The listing builds one solid part. Answer for the finished solid, in the listing's coordinates (mm). A direction names the side the tool comes from. Round coordinates to 2 decimals unless told otherwise and drop trailing zeros. Write each loop counter-clockwise with the first axis right and the second up, starting at its lowest first coordinate (ties: lowest second). Pieces come first, ordered by that corner, then holes. Notation, with made-up numbers: (85.25, 26) - (123.25, 26) arc R21 ccw to (123.25, 56) - close; hole circle Ø5 at (-21, 50.5). An arc over 180 degrees is marked (long way). Answer as CSV lines item,"result". Start each with the question number.
Item 1: For a pull along X with two mould halves and no side action, classify faces 1 (the flat face through (0, -20, 29)), 2 (the cylindrical face through (0, -7.7, 25.5)), 3 (the cylindrical face through (-22.2, -7.7, -12.8)), 4 (the cylindrical face through (32.613, -9.86, 0.018)) as pulls with the +X half, pulls with the -X half, needs draft (parallel to the pull), parting line crosses it, or undercut.
Item 2: A cutting plane is placed at C-C on y = -27. Determine the outline of the cut face in (x, z).
Item 3: Flat-ended cylindrical pins translate along their axes: pin 1 (6 mm diameter, centred on x = 1.5, y = -11.5, fed in from +Z); pin 2 (6.5 mm diameter, centred on y = -3.5, z = -26, fed in from -X); pin 3 (6 mm diameter, centred on y = -6.5, z = -13, fed in from +X). Find the tip coordinate at first contact, or state that the pin passes through.
Item 4: Straight lines are drawn through the part: line 1 along X through (y, z) = (-23.75, 0); line 2 along X through (y, z) = (-18.75, 0); line 3 along Z through (x, y) = (25.5, -14). For each, find the intervals that lie inside material, in ascending order. Write a range as [from, to].
Item 5: A cutting plane is placed at A-A on x = 0. Determine the outline of the cut face in (y, z), and give its area (3 significant figures).
Item 6: A cutting plane is placed at B-B on z = 0. Determine the outline of the cut face in (x, y).
Item 7: Which of the six approach directions +Z, -Z, +X, -X, +Y, -Y give full straight-line access (tool end or side, diameter ignored) to faces 5 (the flat face through (-24.855, -10.14, -14.107)), 6 (the flat face through (-24.645, -10.14, 14.472)), 7 (the conical face through (11.858, -1.995, 20.839)), 8 (the flat face through (21.7, -3.45, 14.82)), 9 (the cylindrical face through (16.291, -9.86, 28.253))?
```python
from build123d import *

# Parameters (mm, degrees)
CUT_EXTRUDE5_START = -20
CUT_EXTRUDE5_DEPTH = 20
FILLET4_R          = 2.5
CUT_EXTRUDE6_START = -86.02405492
CUT_EXTRUDE6_DEPTH = 143.469271841
CIRPATTERN2_COUNT  = 6
CHAMFER1_SIZE      = 3.302
CHAMFER2_SIZE      = 1.27


with BuildPart() as part:
    # Sketch1 → Revolve1 (revolve)
    with BuildSketch(Plane(origin=(0, 0, 0), x_dir=(0, 0, -1), z_dir=(1, 0, 0)), mode=Mode.PRIVATE) as revolve1_sk:
        Polygon((-22.6695, -31.75), (-22.6695, 0), (-33, 0), (-33, -24.619433914), (-25.8445, -31.75), align=None)
    revolve(revolve1_sk.sketch.rotate(Axis((0, 0, 0), (0, 1, 0)), 180), axis=Axis((0, 0, 0), (0, 1, 0)))

    # Sketch4 → Cut-Extrude5 (cut)
    with BuildSketch(Plane(origin=(0, 0, 0), x_dir=(1, 0, 0), z_dir=(0, 1, 0)).offset(CUT_EXTRUDE5_START)):
        with BuildLine():
            ThreePointArc((33, 0), (28.578838325, 16.5), (16.5, 28.578838325))
            Line((16.5, 28.578838325), (33, 0))
        make_face()
        with BuildLine():
            Line((-16.5, 28.578838325), (16.5, 28.578838325))
            ThreePointArc((16.5, 28.578838325), (0, 33), (-16.5, 28.578838325))
        make_face()
        with BuildLine():
            Line((-33, 0), (-16.5, 28.578838325))
            ThreePointArc((-16.5, 28.578838325), (-28.578838325, 16.5), (-33, 0))
        make_face()
        with BuildLine():
            ThreePointArc((16.5, -28.578838325), (28.578838325, -16.5), (33, 0))
            Line((33, 0), (16.5, -28.578838325))
        make_face()
        with BuildLine():
            Line((-16.5, -28.578838325), (-33, 0))
            ThreePointArc((-33, 0), (-28.578838325, -16.5), (-16.5, -28.578838325))
        make_face()
        with BuildLine():
            ThreePointArc((-16.5, -28.578838325), (0, -33), (16.5, -28.578838325))
            Line((16.5, -28.578838325), (-16.5, -28.578838325))
        make_face()
    extrude(amount=CUT_EXTRUDE5_DEPTH, mode=Mode.SUBTRACT)

    # Fillet4
    fillet4_edges = [part.edges().sort_by_distance(p)[0] for p in [
        (33, -10, 0),
        (16.5, -10, -28.578838325),
        (-33, -10, 0),
        (16.5, -10, 28.578838325),
        (-16.5, -10, -28.578838325),
        (-16.5, -10, 28.578838325),
    ]]
    fillet(fillet4_edges, radius=FILLET4_R)

    # Sketch7 → Cut-Extrude6 (cut)
    with BuildSketch(Plane.XY.offset(CUT_EXTRUDE6_START)):
        with BuildLine():
            Line((-1.984375, 0), (-1.984375, -5.715))
            ThreePointArc((-1.984375, -5.715), (0, -7.699375), (1.984375, -5.715))
            Line((1.984375, -5.715), (1.984375, 0))
            Line((1.984375, 0), (0, 0))
            Line((0, 0), (-1.984375, 0))
        make_face()
    cut_extrude6 = extrude(amount=CUT_EXTRUDE6_DEPTH, mode=Mode.SUBTRACT)

    # CirPattern2: Cut-Extrude6 ×6 about axis
    cirpattern2_axis = Axis((0, 0, 0), (0, 1, 0))
    for i in range(1, CIRPATTERN2_COUNT):
        add(cut_extrude6.rotate(cirpattern2_axis, i * 360 / CIRPATTERN2_COUNT), mode=Mode.SUBTRACT)

    # Chamfer1
    chamfer1_edges = [part.edges().sort_by_distance(p)[0] for p in [
        (-11.33475, 0, 19.632362891),
        (-22.6695, 0, 0),
        (-11.33475, 0, -19.632362891),
        (22.6695, 0, 0),
        (11.33475, 0, 19.632362891),
        (11.33475, 0, -19.632362891),
    ]]
    chamfer(chamfer1_edges, length=CHAMFER1_SIZE)

    # Chamfer2
    chamfer2_edges = [part.edges().sort_by_distance(p)[0] for p in [
        (0, -31.75, 22.6695),
    ]]
    chamfer(chamfer2_edges, length=CHAMFER2_SIZE)


solid = part.part
```
Geometry says:
1,face 1,"needs draft"
1,face 2,"undercut"
1,face 3,"undercut"
1,face 4,"pulls with the +X half"
2,outline,"circle Ø61.22 at (0, 0); hole circle Ø45.34 at (0, 0)"
3,pin 1,"stops at z = 28.58"
3,pin 2,"stops at x = -19.87"
3,pin 3,"stops at x = 27.23"
4,line 1,"x = [-33, -22.67], [22.67, 33]"
4,line 2,"x = [-32.61, -22.67], [22.67, 32.61]"
4,line 3,"z = [-12.99, 12.99]"
5,outline,"(-31.75, -25.84) - (-24.62, -33) - (-20, -33) - (-20, -28.58) - (-7.7, -28.58) - (-7.7, -22.67) - (-30.48, -22.67) - (-31.75, -23.94) - close; (-31.75, 23.94) - (-30.48, 22.67) - (-7.7, 22.67) - (-7.7, 28.58) - (-20, 28.58) - (-20, 33) - (-24.62, 33) - (-31.75, 25.84) - close"
5,area,"336 mm^2"
6,outline,"(-33, -24.62) - (-25.84, -31.75) - (-23.94, -31.75) - (-22.67, -30.48) - (-22.67, -3.3) - (-25.97, 0) - (-32.61, 0) - (-32.61, -20) - (-33, -20) - close; (22.67, -30.48) - (23.94, -31.75) - (25.84, -31.75) - (33, -24.62) - (33, -20) - (32.61, -20) - (32.61, 0) - (25.97, 0) - (22.67, -3.3) - close"
7,face 5,"-Z, -X, +Y"
7,face 6,"+Z, -X, +Y"
7,face 7,"+Y"
7,face 8,"+X, +Y"
7,face 9,"+Z, +X, +Y"
